Autodesk Inventor part; units mm, degrees
ref_plane "YZ Plane" through (0, 0, 0) normal (1, 0, 0) x (0, 1, 0)
ref_plane "XZ Plane" through (0, 0, 0) normal (0, 1, 0) x (-1, 0, 0)
ref_plane "XY Plane" through (0, 0, 0) normal (0, 0, 1) x (1, 0, 0)
sketch "Sketch1" plane through (0, 0, 0) normal (0, 0, 1) x (1, 0, 0)
  line L0 (-11, 5.5) -> (11, 5.5)
  line L1 (11, 5.5) -> (11, -5.5)
  line L2 (11, -5.5) -> (-11, -5.5)
  line L3 (-11, -5.5) -> (-11, 5.5)
  line L4 (-11, 5.5) -> (11, -5.5) construction
  line L5 (11, 5.5) -> (-11, -5.5) construction
  point P0 (0, 0)
  dimension "d0" = 22
  dimension "d1" = 11
extrude "Extrusion1" add sketch "Sketch1" along normal blind 9
sketch "Sketch2" plane through (-11, 5.5, 0) normal (0, 1, 0) x (1, 0, 0)
  line L0 (0, 0) -> (0, -9)
  line L1 (22, 0) -> (22, -9)
  circle A0 centre (4, -5) radius 1.5
  circle A1 centre (18, -5) radius 1.5
  line L2 (0, 0) -> (22, 0)
  line L3 (22, 0) -> (22, -9)
  line L4 (4, 0) -> (4, -5)
  line L5 (18, -5) -> (18, 0)
  line L6 (0, -5) -> (4, -5)
  line L7 (22, -5) -> (18, -5)
  point P0 (11, 0)
  point P1 (9, -4)
  dimension "d6" = 3
  dimension "d7" = 3
  dimension "d25" = 5
  dimension "d26" = 5
  dimension "d27" = 4
  dimension "d28" = 4
extrude "Extrusion2" cut sketch "Sketch2" against normal up to next contours L6 L4 A0 | A0 L4 L6 | L5 L7 A1 | A1 L7 L5
sketch "Sketch3" plane through (11, -5.5, 0) normal (1, 0, 0) x (0, 0, -1)
  line L0 (-9, 0) -> (-9, 11)
  line L1 (0, 0) -> (-9, 0)
  line L2 (-9, 11) -> (-9, 0)
  line L3 (-9, 11) -> (-9, 0)
  arc A0 (-9, -0.0647) -> (-9, 11) centre (-18.452, 5.4676) ccw
  line L4 (-9, 11) -> (-9, -0.0647)
  line L5 (-6.5, 11) -> (-6.5, 0)
  line L6 (0, 0) -> (0, 11)
  line L7 (0, 6.25) -> (0, 4.75)
  point P0 (0, 5.5)
extrude "Extrusion3" cut sketch "Sketch3" against normal up to next
sketch "Sketch6" plane through (0, 0, 0) normal (0, 0, -1) x (-1, 0, 0)
  line L0 (-11, 5.5) -> (-11, -5.5)
  line L1 (-11, 5.5) -> (-11, 2.5)
  line L2 (-11, -5.5) -> (11, -5.5)
  line L3 (-11, -5.5) -> (-11, -2.5)
  line L4 (0, 0) -> (0, -2)
  line L5 (0, -2) -> (9, -2)
  line L6 (0, 0) -> (0, 2)
  line L7 (0, 2) -> (-9, 2)
  line L8 (9, -2) -> (-9, -2)
  line L9 (-9, -2) -> (-9, 2)
  line L10 (-9, 2) -> (9, 2)
  line L11 (9, 2) -> (9, -2)
  line L12 (-11, -5.5) -> (11, -5.5)
  line L13 (11, -5.5) -> (11, 5.5)
  dimension "d40" = 2
  dimension "d41" = 9
  dimension "d42" = 2
  dimension "d43" = 9
extrude "Extrusion6" cut sketch "Sketch6" against normal blind 5
sketch "Sketch4" plane through (-11, -5.5, 0) normal (0, -1, 0) x (1, 0, 0)
  line L0 (11, 0) -> (11, 2.5)
  line L1 (0, 0) -> (22, 0)
  line L2 (12.5, 5) -> (9.5, 5)
  line L3 (9.5, 5) -> (9.5, 0)
  line L4 (9.5, 0) -> (12.5, 0)
  line L5 (12.5, 0) -> (12.5, 5)
  line L6 (12.5, 5) -> (9.5, 0) construction
  line L7 (9.5, 5) -> (12.5, 0) construction
  line L8 (22, 8.9624) -> (0, 8.9624)
  line L9 (12.5, 5) -> (15, 5)
  line L10 (15, 5) -> (15, 8.9624)
  line L11 (9.5, 5) -> (7, 5)
  line L12 (7, 5) -> (7, 9)
  line L13 (22, 9) -> (0, 9)
  line L14 (7, 9) -> (15, 8.9624)
  dimension "d13" = 2.5
  dimension "d14" = 3
  dimension "d34" = 2.5
  dimension "d35" = 2.5
extrude "Extrusion4" cut sketch "Sketch4" against normal up to surface (3.5 mm away)
sketch "Sketch5" plane through (11, -5.5, 0) normal (1, 0, 0) x (0, 0, -1)
  line L0 (0, 5.5) -> (-4, 5.5)
  line L1 (-5, 0) -> (-5, 3)
  line L2 (0, 5.5) -> (0, 4.75)
  line L3 (0, 0) -> (0, 11)
  line L4 (-4, 5.5) -> (-4, 6.25)
  line L5 (0, 4.75) -> (-4, 4.75)
  line L6 (-4, 4.75) -> (-4, 6.25)
  line L7 (-4, 6.25) -> (0, 6.25)
  line L8 (0, 6.25) -> (0, 4.75)
  point P0 (-5, 11)
  dimension "d20" = 4
  dimension "d21" = 0.75
  dimension "d22" = 0.75
extrude "Extrusion5" cut sketch "Sketch5" against normal up to next
ref_plane "Work Plane1" through (11, 0, 0) normal (0, -1, 0) x (1, 0, 0)
mirror "Mirror1" about plane through (11, 0, 0) normal (0, -1, 0) of "Extrusion4"
equation "\"d7\" = d6"
equation "\"d26\" = d25"
equation "\"d28\" = d27"
equation "\"d22\" = d21"
properties part number "back_pack_clip_in_2"
Work out the finished part from the listing and answer in its coordinate system (mm). A direction names the side the tool comes from. Round coordinates to 2 decimals unless told otherwise and drop trailing zeros. Order: outer loops, then holes, each group sorted by start corner. A loop starts at its lowest first (then second) coordinate and runs counter-clockwise, first axis right, second up. Notation, with made-up numbers: M 2,27.5 L 47,27.5 A29 cw 47,65.5 Z; hole C 27,50 d9. An arc over 180 degrees is marked long. One line per item, written item: value.
Q1. Find section D-D on z = 4.5. Give the number of separate pieces and of enclosed holes in the cut face, then the cut area to 3 significant figures.
Derived:
separate pieces: 6
enclosed holes: 0
area: 109 mm²
Q2. Flat-ended cylindrical pins translate along their axes: pin 1 (2 mm diameter, centred on x = -2, y = 2, fed in from +Z); pin 2 (3 mm diameter, centred on x = 0.5, z = 6.5, fed in from -Y). Find the tip coordinate at first contact, or state that the pin passes through.
Derived:
pin 1: z = 7.69
pin 2: y = -2
Q3. For faces 4 (the face through (0, 2, 6)), 5 (the face through (-5, 2, 2)), 6 (the face through (4, -4, 7)), 7 (the face through (-1.5, 4, 2)), determine the directions among +Z, -Z, +X, -X, +Y, -Y from which every point of the face is accessible in a straight line to the end or side of a thin tool.
Derived:
face 4: +Z, +Y
face 5: -Z
face 6: +Z, -Y
face 7: +Z, -Z, +Y, -Y
Q4. Find section A-A on z = 1.5. Write down the section's boundary in (x, y), then the cut area to 3 significant figures.
Derived:
outline: M -11,-5.5 L -1.5,-5.5 L -1.5,-2 L -9,-2 L -9,2 L -1.5,2 L -1.5,5.5 L -11,5.5 Z; M 1.5,-5.5 L 11,-5.5 L 11,-0.75 L 9,-0.75 L 9,-2 L 1.5,-2 Z; M 1.5,2 L 9,2 L 9,0.75 L 11,0.75 L 11,5.5 L 1.5,5.5 Z
area: 146 mm²
Q5. Find section C-C on y = 4.75. Write down the section's boundary in (x, z).
Derived:
outline: M -11,0 L -1.5,0 L -1.5,5 L -4,5 L -4,8.6 L -11,8.6 Z; M 1.5,0 L 11,0 L 11,8.6 L 4,8.6 L 4,5 L 1.5,5 Z; hole C -7,5 d3; hole C 7,5 d3
Q6. Straight lines are drawn through the part: line 1 (Y direction, x = 3.75, z = 1.5); line 2 (X direction, y = 4, z = 5.5); line 3 (Y direction, x = -0.5, z = 5.75). For each, find the intervals that lie inside material, in ascending order.
Derived:
line 1: -5.5 to -2, 2 to 5.5
line 2: -11 to -8.41, -5.59 to -4, 4 to 5.59, 8.41 to 11
line 3: -2 to 2
Q7. Determine the mould class of faces 1 (the face through (-11, 0, 4)), 2 (the face through (6, -4, 0)), 3 (the face through (-5, -2, 2)) for opening direction X: released by +X, released by -X, zero draft, split by the parting line, or undercut.
Derived:
face 1: released by -X
face 2: zero draft
face 3: undercut
Q8. Find section B-B on x = 7. Write down the section's boundary in (y, z), then the cut area to 3 significant figures.
Derived:
outline: M -5.5,0 L -2,0 L -2,3.5 L -5.5,3.5 Z; M -5.5,6.5 L 5.5,6.5 L 5.5,9 A10.95 cw -5.5,8.96 Z; M 2,0 L 5.5,0 L 5.5,3.5 L 2,3.5 Z
area: 40.8 mm²
